from build123d import *

# Parameters (mm, degrees)
SKETCH1_W           = 139.5
SKETCH1_H           = 152.4
BOSS_EXTRUDE1_DEPTH = 6.35
SKETCH2_W           = 139.5
SKETCH2_H           = 152.4
CUT_EXTRUDE1_DEPTH  = 3.375
SKETCH3_R           = 2.286
BOSS_EXTRUDE2_DEPTH = 12.7
SKETCH4_R           = 2.286
BOSS_EXTRUDE3_DEPTH = 12.7
SKETCH5_R           = 4.191
CUT_EXTRUDE2_DEPTH  = 16.675000158


with BuildPart() as part:
    # Sketch1 → Boss-Extrude1 (new body)
    with BuildSketch(Plane(origin=(0, 0, 0), x_dir=(1, 0, 0), z_dir=(0, 1, 0))):
        with Locations((69.75, 76.2)):
            Rectangle(SKETCH1_W, SKETCH1_H)
    extrude(amount=BOSS_EXTRUDE1_DEPTH)

    # Sketch2 → Cut-Extrude1 (cut)
    with BuildSketch(Plane(origin=(0, 6.35, 0), x_dir=(1, 0, 0), z_dir=(0, 1, 0))):
        with Locations((69.75, 76.2)):
            Rectangle(SKETCH2_W, SKETCH2_H)
    extrude(amount=-CUT_EXTRUDE1_DEPTH, mode=Mode.SUBTRACT)

    # Sketch3 → Boss-Extrude2 (add)
    with BuildSketch(Plane.XY):
        with BuildLine():
            Line((63.4, 9.325), (63.4, 2.975))
            Line((63.4, 2.975), (76.1, 2.975))
            Line((76.1, 2.975), (76.1, 9.325000158))
            ThreePointArc((76.1, 9.325000158), (69.749999921, 15.675000158), (63.4, 9.325))
        make_face()
        with Locations((69.75, 9.325000158)):
            Circle(SKETCH3_R, mode=Mode.SUBTRACT)
    extrude(amount=-BOSS_EXTRUDE2_DEPTH)

    # Sketch4 → Boss-Extrude3 (add)
    with BuildSketch(Plane(origin=(0, 0, -152.4), x_dir=(-1, 0, 0), z_dir=(0, 0, -1))):
        with BuildLine():
            Line((-130.61, 9.325), (-130.61, 2.975))
            Line((-130.61, 2.975), (-117.91, 2.975))
            Line((-117.91, 2.975), (-117.91, 9.325))
            ThreePointArc((-117.91, 9.325), (-124.26, 15.675), (-130.61, 9.325))
        make_face()
        with Locations((-124.26, 9.325)):
            Circle(SKETCH4_R, mode=Mode.SUBTRACT)
        with BuildLine():
            Line((-21.59, 9.325), (-21.59, 2.975))
            Line((-21.59, 2.975), (-8.89, 2.975))
            Line((-8.89, 2.975), (-8.89, 9.325))
            ThreePointArc((-8.89, 9.325), (-15.24, 15.675), (-21.59, 9.325))
        make_face()
        with Locations((-15.24, 9.325)):
            Circle(SKETCH4_R, mode=Mode.SUBTRACT)
    extrude(amount=-BOSS_EXTRUDE3_DEPTH)

    # Sketch5 → Cut-Extrude2 (cut, through all)
    with BuildSketch(Plane.XZ):
        with Locations((33.274, -136.991598)):
            Circle(SKETCH5_R)
    extrude(amount=-CUT_EXTRUDE2_DEPTH, mode=Mode.SUBTRACT)


solid = part.part
Input: part model. Units: mm. Frame: model coordinates. A direction names the side the tool comes from. Coordinates: 2 decimals unless noted, no trailing zeros. Loops run counter-clockwise (first coordinate to the right, second up) from the corner with the lowest first, then second, coordinate; pieces in that order, holes last.
(1) Section C-C on x = 86. Return the cut outline in (y, z) (3 decimals), then the cut area to 3 significant figures.
(2) Set-up query: faces 5 (the face through (69, 2, -152.4)), 6 (the face through (8.89, 6, -146)), 7 (the face through (130.61, 6, -146)), 8 (the face through (117.91, 6, -146)), 9 (the face through (124.3, 6.6, -139.7)). Return all of +Z, -Z, +X, -X, +Y, -Y with unobstructed straight access to the full face (end or side cutting, diameter ignored); none if empty.
(3) Section B-B on z = -37.5. Return the cut outline in (x, y) (3 decimals), then the cut area to 3 significant figures.
(4) Pull-direction query (Y, two-part tool) for faces 1 (the face through (68.065, 10.87, -6.261)), 2 (the face through (13.13, 8.45, -146.14)), 3 (the face through (69, 0, -77)), 4 (the face through (69, 4, 0)); classes: released by +Y, released by -Y, zero draft, split by the parting line, or undercut.
(5) Section A-A on x = 69.75. Return the cut outline in (y, z) (3 decimals).
(6) Material intervals for probe 1 along Y at (x, z) = (15.24, -148.5) (3 decimals); probe 2 along Y at (x, z) = (7, -116) (3 decimals); probe 3 along Z at (x, y) = (16.5, 6.75), sorted ascending.
(7) First-contact query: pin 1 Ø1.9 at (y, z) = (5.5, -145.5) entering from -X; pin 2 Ø4 at (x, y) = (123.5, 8.5) entering from +Z; pin 3 Ø10 at (x, z) = (75, -43) entering from -Y; pin 4 Ø3 at (x, y) = (75, 7) entering from -Z. Flat tips, straight axial feed; report the tip coordinate or a pass-through.
Data:
1. outline: (0, -152.4) - (2.975, -152.4) - (2.975, 0) - (0, 0) - close
1. area: 453 mm2
2. face 5: -Z, +X, -X, +Y, -Y
2. face 6: +Z, -Z, -X, +Y
2. face 7: +Z, -Z, +X, +Y
2. face 8: +Z, -Z, +Y
2. face 9: +Z, +X, -X, +Y
3. outline: (0, 0) - (139.5, 0) - (139.5, 2.975) - (0, 2.975) - close
3. area: 415 mm2
4. face 1: undercut
4. face 2: undercut
4. face 3: released by -Y
4. face 4: zero draft
5. outline: (0, -152.4) - (2.975, -152.4) - (2.975, -12.7) - (7.039, -12.7) - (7.039, 0) - (0, 0) - close; (11.611, -12.7) - (15.675, -12.7) - (15.675, 0) - (11.611, 0) - close
6. probe 1: y = 0 to 7.039, 11.611 to 15.675
6. probe 2: y = 0 to 2.975
6. probe 3: z = -152.4 to -139.7
7. pin 1: stops at x = 8.89
7. pin 2: stops at z = -139.7
7. pin 3: stops at y = 0
7. pin 4: stops at z = -12.7
